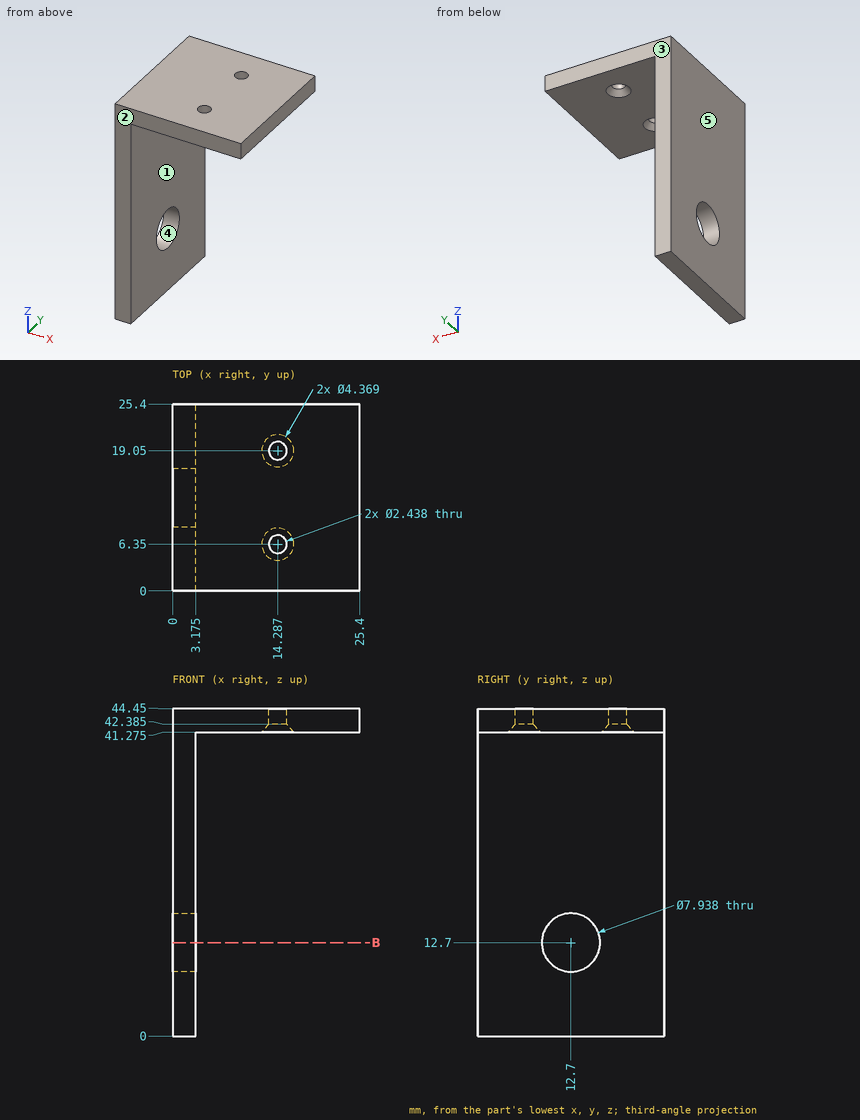
Print and shaded views of the part. All mm, measured from the part's lowest x, y and z. A direction names the side the tool comes from. Coordinates: 2 decimals unless noted, no trailing zeros. Loops run counter-clockwise (first coordinate to the right, second up) from the corner with the lowest first, then second, coordinate; pieces in that order, holes last. Notation, with made-up numbers: M -32.5,34.5 L 24.5,34.5 A19 ccw 24.5,44.5 Z; hole C 9.25,77.5 d6. An arc over 180 degrees is marked long. Use a Markdown table: item, result. Add a question column.
Q1. Pin check, flat tips, straight feed: P1, Ø2, axis at x = 14.29, y = 6.35, coming from the +Z side; P2, Ø11, axis at x = 14, y = 9, coming from the -Z side (1 decimal). Stop position of each tip, or through.
Q2. Probe L1, parallel to Y at x = 2.5, z = 12.7; L2, parallel to X at y = 6.35, z = 43.3; L3, parallel to X at y = 6, z = 13 (1 decimal). List the from-to ranges inside material, lowest first.
Q3. Mould opens along Y. For the marked faces 3, 4 and 5 say: +Y half, -Y half, draft (parallel to the pull), parting line (faces both ways), or undercut.
Q4. Cut at B-B (z = 12.7). Write the cut outline in (x, y) (1 decimal).
Q5. Which spindle directions (+Z, -Z, +X, -X, +Y, -Y) get a long thin tool onto all of the face, cutting with end or side? Do the marked faces 1 and 2. Say none if no direction does.
Worked out:
| question | item | result |
|---|---|---|
| 1 | P1 | passes through |
| 1 | P2 | stops at z = 41.3 |
| 2 | L1 | y = 0 to 8.73, 16.67 to 25.4 |
| 2 | L2 | x = 0 to 13.07, 15.51 to 25.4 |
| 2 | L3 | x = 0 to 3.2 |
| 3 | face 3 | +Y half |
| 3 | face 4 | undercut |
| 3 | face 5 | draft |
| 4 | outline | M 0,0 L 3.2,0 L 3.2,8.7 L 0,8.7 Z; M 0,16.7 L 3.2,16.7 L 3.2,25.4 L 0,25.4 Z |
| 5 | face 1 | -Z, +X, +Y, -Y |
| 5 | face 2 | +Z, -Z, +X, -X, -Y |
